The listing builds one solid part. Answer for the finished solid, in the listing's coordinates (mm). A direction names the side the tool comes from. Give positions to 0.01 mm unless a question says otherwise; leave off trailing zeros. Loops run counter-clockwise (first coordinate to the right, second up) from the corner with the lowest first, then second, coordinate; pieces in that order, holes last. Notation, with made-up numbers: M 18.25,-7 L 35.25,-7 A23 cw 35.25,32 Z; hole C -19.75,73.25 d9. An arc over 180 degrees is marked long. One line per item, written item: value. Start each with the question number.
Q1. A cutting plane is placed at C-C, the plane y = 30. Determine the outline of the cut face in (x, z) (3 decimals), and give its area (3 significant figures).
Q2. Flat-ended cylindrical pins translate along their axes: pin 1 (3 mm diameter, centred on x = 8, z = 6, fed in from +Y); pin 2 (3 mm diameter, centred on x = 3.5, y = -5.5, fed in from +Z); pin 3 (10 mm diameter, centred on x = 11, z = 2.5, fed in from -Y); pin 4 (6 mm diameter, centred on x = 4, z = 17.5, fed in from +Y). Find the tip coordinate at first contact, or state that the pin passes through.
Q3. A cutting plane is placed at D-D, the plane z = 8.75. Determine the outline of the cut face in (x, y) (3 decimals), and give its area (3 significant figures).
Q4. A cutting plane is placed at A-A, the plane x = 0. Determine the outline of the cut face in (y, z) (3 decimals), and give its area (3 significant figures).
Q5. For faces 1 (the flat face through (0, -50, 1)), 2 (the cylindrical face through (-0.69, 26.9, 12.86)), determine the directions among +Z, -Z, +X, -X, +Y, -Y from which every point of the face is accessible in a straight line to the end or side of a thin tool.
Q6. A cutting plane is placed at B-B, the plane z = 1.75. Determine the outline of the cut face in (x, y) (3 decimals), and give its area (3 significant figures).
Q7. Consider L1, parallel to Y at x = 0, z = 2.2 (3 decimals); L2, parallel to Z at x = 10, y = -19.5; L3, parallel to Y at x = 2, z = 15.75. Determine where each line is inside the solid, lowest interval first.
from build123d import *

# Parameters (mm, degrees)
CROQUIS1_R              = 3.175
SALIENTE_EXTRUIR1_DEPTH = 3
CROQUIS2_R              = 3.175
SALIENTE_EXTRUIR2_DEPTH = 20


with BuildPart() as part:
    # Croquis1 → Saliente-Extruir1 (new body)
    with BuildSketch(Plane.XY):
        with BuildLine():
            Line((5, -50), (-5, -50))
            ThreePointArc((-5, -50), (-12.071067812, -47.071067812), (-15, -40))
            Line((-15, -40), (-15, 40))
            ThreePointArc((-15, 40), (-12.071067812, 47.071067812), (-5, 50))
            Line((-5, 50), (5, 50))
            ThreePointArc((5, 50), (12.071067812, 47.071067812), (15, 40))
            Line((15, 40), (15, -40))
            ThreePointArc((15, -40), (12.071067812, -47.071067812), (5, -50))
        make_face()
        with Locations((0, -40)):
            Circle(CROQUIS1_R, mode=Mode.SUBTRACT)
    extrude(amount=SALIENTE_EXTRUIR1_DEPTH)

    # Croquis2 → Saliente-Extruir2 (add)
    with BuildSketch(Plane.XY.offset(3)):
        with Locations((0, 30)):
            Circle(CROQUIS2_R)
    extrude(amount=SALIENTE_EXTRUIR2_DEPTH)


solid = part.part
Answer block:
1. outline: M -15,0 L 15,0 L 15,3 L 3.175,3 L 3.175,23 L -3.175,23 L -3.175,3 L -15,3 Z
1. area: 217 mm^2
2. pin 1: through
2. pin 2: z = 3
2. pin 3: y = -49.95
2. pin 4: y = 33.01
3. outline: C 0,30 d6.35
3. area: 31.7 mm^2
4. outline: M -50,0 L -43.175,0 L -43.175,3 L -50,3 Z; M -36.825,0 L 50,0 L 50,3 L 33.175,3 L 33.175,23 L 26.825,23 L 26.825,3 L -36.825,3 Z
4. area: 408 mm^2
5. face 1: +Z, -Z, +X, -X, -Y
5. face 2: +Z
6. outline: M -15,-40 A10 ccw -5,-50 L 5,-50 A10 ccw 15,-40 L 15,40 A10 ccw 5,50 L -5,50 A10 ccw -15,40 Z; hole C 0,-40 d6.35
6. area: 2,880 mm^2
7. L1: -50 to -43.175, -36.825 to 50
7. L2: 0 to 3
7. L3: 27.53 to 32.47
